from build123d import *

# Parameters (mm, degrees)
F1_DEPTH        = 1
F1_COPIES_COUNT = 10
F3_W            = 3
F3_H            = 3
F4_DEPTH        = 0.25
F5_DEPTH        = 1
F6_DEPTH        = 0.25
F7_R            = 1.1
F8_DEPTH        = 12.5


# Not quite as in the source:
# - ends of sketch curves that miss each other by under 0.0002 mm in the source are joined
# - a feature of the source that left no trace in its solid (it failed there, or was rolled back) is left out
# - a pattern or mirror of a feature is missing from the dataset's text; its kind, count and spacing are read off the source's solid


with BuildPart() as f1:
    # F0 (on Top) → F1 (new body)
    with BuildSketch(Plane.XY):
        with BuildLine():
            ThreePointArc((0.581444512, 2.1217733808), (0.2933415776, 2.1803556405), (0, 2.2))
            ThreePointArc((0, 2.2), (-0.2933416878, 2.1803556256), (-0.5814447265, 2.121773322))
            ThreePointArc((-0.5814447265, 2.121773322), (-0.5968372157, 2.1167523736), (-0.6125853979, 2.1129929319))
            ThreePointArc((-0.6125853979, 2.1129929319), (-1.3214219849, -1.7589326132), (2.2, 0))
            ThreePointArc((2.2, 0), (1.7589325969, 1.3214220066), (0.612585346, 2.112992947))
            ThreePointArc((0.6125853416, 2.1129929319), (0.5968370782, 2.1167523965), (0.581444512, 2.1217733808))
        make_face()
        with BuildLine():
            ThreePointArc((0.6, 0.8), (0, -1), (-0.6, 0.8))
            Line((-0.6, 0.8), (0, 0.8))
            Line((0, 0.8), (0.6, 0.8))
        make_face(mode=Mode.SUBTRACT)
        with BuildLine():
            ThreePointArc((-0.5814447265, 2.121773322), (-0.2933416878, 2.1803556256), (0, 2.2))
            Line((0, 2.2), (0, 2.8273255734))
            ThreePointArc((0, 2.8273255734), (-0.1215931939, 2.889819495), (-0.1419835484, 3.0250031792))
            Line((-0.1419835484, 3.0250031792), (-0.4660251262, 2.233467269))
            ThreePointArc((-0.4660251262, 2.233467269), (-0.5120300634, 2.1655250062), (-0.5814447265, 2.121773322))
        make_face()
        with BuildLine():
            Line((0, 2.8273255734), (0, 2.2))
            ThreePointArc((0, 2.2), (0.2933415776, 2.1803556405), (0.581444512, 2.1217733808))
            ThreePointArc((0.581444512, 2.1217733808), (0.5119904355, 2.165563311), (0.4659834267, 2.2335690598))
            Line((0.4659834267, 2.2335690598), (0.1424618925, 3.0249932315))
            ThreePointArc((0.1424618925, 3.0249932315), (0.1482808399, 3.0014743175), (0.1502375048, 2.9773253853))
            ThreePointArc((0.1502375048, 2.9773253853), (0.1062195181, 2.8711754307), (0, 2.8273255734))
        make_face()
        with BuildLine():
            ThreePointArc((-0.1419835484, 3.0250031792), (-0.1215931939, 2.889819495), (0, 2.8273255734))
            Line((0, 2.8273255734), (0, 3.1273251973))
            ThreePointArc((0, 3.1273251973), (-0.0874611784, 3.0990173775), (-0.1419835484, 3.0250031792))
        make_face()
        with BuildLine():
            Line((0, 3.1273251973), (0, 2.8273255734))
            ThreePointArc((0, 2.8273255734), (0.1062195181, 2.8711754307), (0.1502375048, 2.9773253853))
            ThreePointArc((0.1502375048, 2.9773253853), (0.1482808399, 3.0014743175), (0.1424618925, 3.0249932315))
            ThreePointArc((0.1424618925, 3.0249932315), (0.0877476558, 3.0991530237), (0, 3.1273251973))
        make_face()
        with BuildLine():
            ThreePointArc((0.612585346, 2.112992947), (0.5970310708, 2.1174404125), (0.581444512, 2.1217733808))
            ThreePointArc((0.581444512, 2.1217733808), (0.5968370782, 2.1167523965), (0.6125853416, 2.1129929319))
        make_face()
        with BuildLine():
            ThreePointArc((-0.6125853979, 2.1129929319), (-0.5968372157, 2.1167523736), (-0.5814447265, 2.121773322))
            ThreePointArc((-0.5814447265, 2.121773322), (-0.5970312038, 2.117440375), (-0.6125853979, 2.1129929319))
        make_face()
    extrude(amount=F1_DEPTH)

    # F1_copies: F1 ×10 about axis
    f1_copies_axis = Axis((0, 0, 0), (0, 0, 1))


with BuildPart() as f1_1:
    add(f1.part)
    for i in range(1, F1_COPIES_COUNT):
        add(f1.part.rotate(f1_copies_axis, i * 360 / F1_COPIES_COUNT))

    # F3 (on face) → F4 (cut)
    with BuildSketch(Plane.XY.offset(1)):
        Rectangle(F3_W, F3_H)
    extrude(amount=-F4_DEPTH, mode=Mode.SUBTRACT)

    # F0 (on Top) → F5 (join)
    with BuildSketch(Plane.XY):
        with BuildLine():
            ThreePointArc((0.581444512, 2.1217733808), (0.2933415776, 2.1803556405), (0, 2.2))
            ThreePointArc((0, 2.2), (-0.2933416878, 2.1803556256), (-0.5814447265, 2.121773322))
            ThreePointArc((-0.5814447265, 2.121773322), (-0.5968372157, 2.1167523736), (-0.6125853979, 2.1129929319))
            ThreePointArc((-0.6125853979, 2.1129929319), (-1.3214219849, -1.7589326132), (2.2, 0))
            ThreePointArc((2.2, 0), (1.7589325969, 1.3214220066), (0.612585346, 2.112992947))
            ThreePointArc((0.6125853416, 2.1129929319), (0.5968370782, 2.1167523965), (0.581444512, 2.1217733808))
        make_face()
        with BuildLine():
            ThreePointArc((0.6, 0.8), (0, -1), (-0.6, 0.8))
            Line((-0.6, 0.8), (0, 0.8))
            Line((0, 0.8), (0.6, 0.8))
        make_face(mode=Mode.SUBTRACT)
        with BuildLine():
            ThreePointArc((-0.5814447265, 2.121773322), (-0.2933416878, 2.1803556256), (0, 2.2))
            Line((0, 2.2), (0, 2.8273255734))
            ThreePointArc((0, 2.8273255734), (-0.1215931939, 2.889819495), (-0.1419835484, 3.0250031792))
            Line((-0.1419835484, 3.0250031792), (-0.4660251262, 2.233467269))
            ThreePointArc((-0.4660251262, 2.233467269), (-0.5120300634, 2.1655250062), (-0.5814447265, 2.121773322))
        make_face()
        with BuildLine():
            Line((0, 2.8273255734), (0, 2.2))
            ThreePointArc((0, 2.2), (0.2933415776, 2.1803556405), (0.581444512, 2.1217733808))
            ThreePointArc((0.581444512, 2.1217733808), (0.5119904355, 2.165563311), (0.4659834267, 2.2335690598))
            Line((0.4659834267, 2.2335690598), (0.1424618925, 3.0249932315))
            ThreePointArc((0.1424618925, 3.0249932315), (0.1482808399, 3.0014743175), (0.1502375048, 2.9773253853))
            ThreePointArc((0.1502375048, 2.9773253853), (0.1062195181, 2.8711754307), (0, 2.8273255734))
        make_face()
        with BuildLine():
            ThreePointArc((-0.1419835484, 3.0250031792), (-0.1215931939, 2.889819495), (0, 2.8273255734))
            Line((0, 2.8273255734), (0, 3.1273251973))
            ThreePointArc((0, 3.1273251973), (-0.0874611784, 3.0990173775), (-0.1419835484, 3.0250031792))
        make_face()
        with BuildLine():
            Line((0, 3.1273251973), (0, 2.8273255734))
            ThreePointArc((0, 2.8273255734), (0.1062195181, 2.8711754307), (0.1502375048, 2.9773253853))
            ThreePointArc((0.1502375048, 2.9773253853), (0.1482808399, 3.0014743175), (0.1424618925, 3.0249932315))
            ThreePointArc((0.1424618925, 3.0249932315), (0.0877476558, 3.0991530237), (0, 3.1273251973))
        make_face()
        with BuildLine():
            ThreePointArc((0.612585346, 2.112992947), (0.5970310708, 2.1174404125), (0.581444512, 2.1217733808))
            ThreePointArc((0.581444512, 2.1217733808), (0.5968370782, 2.1167523965), (0.6125853416, 2.1129929319))
        make_face()
        with BuildLine():
            ThreePointArc((-0.6125853979, 2.1129929319), (-0.5968372157, 2.1167523736), (-0.5814447265, 2.121773322))
            ThreePointArc((-0.5814447265, 2.121773322), (-0.5970312038, 2.117440375), (-0.6125853979, 2.1129929319))
        make_face()
    extrude(amount=F5_DEPTH)

    # F3 (on face) → F6 (join)
    with BuildSketch(Plane.XY.offset(1)):
        Rectangle(F3_W, F3_H)
        Polygon((-0.259935757, 0.8), (0.259935757, 0.8), (0.6805206467, 0.494427191), (0.8411697794, 0), (0.6805206467, -0.494427191), (0.259935757, -0.8), (-0.259935757, -0.8), (-0.6805206467, -0.494427191), (-0.8411697794, 0), (-0.6805206467, 0.494427191), align=None, mode=Mode.SUBTRACT)
    extrude(amount=F6_DEPTH)

    # F7 (on face) → F8 (cut, symmetric)
    with BuildSketch(Plane.XY.offset(1)):
        Circle(F7_R)
    extrude(amount=F8_DEPTH, both=True, mode=Mode.SUBTRACT)


solid = f1_1.part
Could you check a few things on this model? Use its own coordinates, in mm. A direction names the side the tool comes from. Give positions to 0.01 mm unless a question says otherwise; leave off trailing zeros. Order: outer loops, then holes, each group sorted by start corner. A loop starts at its lowest first (then second) coordinate and runs counter-clockwise, first axis right, second up. Notation, with made-up numbers: (49, 68) -> (96, 68) arc R11 ccw to (96, 81) -> close; hole circle Ø9 at (56, -28). An arc over 180 degrees is marked (long way). Return JSON: item names as keys, results as strings.
1. Thinking about a two-plate mould opening in Y: for faces 4 (the flat face through (2.41, 1.1, 0.49)), 5 (the flat face through (-1, -1, 0)), 6 (the flat face through (-1.79, -1.94, 0.49)), which applies, pulls with the +Y half, pulls with the -Y half, needs draft (parallel to the pull), parting line crosses it, or undercut?
Answer list:
{"face 4": "pulls with the +Y half", "face 5": "needs draft", "face 6": "undercut"}
2. Imagine slicing it at A-A on x = 2.6. List the corners of the cut face in (y, z) for me, then the cut area to 3 significant figures.
Answer list:
{"outline": "(-1.09, 0) -> (-0.53, 0) -> (-0.53, 1) -> (-1.09, 1) -> close; (0.53, 0) -> (1.09, 0) -> (1.09, 1) -> (0.53, 1) -> close", "area": "1.12 mm2"}
3. For pin 1 Ø1.8 at (x, y) = (0, 0) entering from -Z, with a flat end and sliding along its axis, tell me the tip position at first contact or that it passes through.
Answer list:
{"pin 1": "passes through"}
4. Imagine slicing it at B-B on y = 2.75. List the corners of the cut face in (x, z) for me.
Answer list:
{"outline": "(-0.25, 0) -> (0.25, 0) -> (0.25, 1) -> (-0.25, 1) -> close"}
5. On a 3-axis mill with a long thin cutter (end or side, diameter ignored), from which of +Z, -Z, +X, -X, +Y, -Y can I reach the whole of each face in a straight line? I mean faces 1 (the cylindrical face through (1.05, 0.33, 0.63)), 2 (the flat face through (1.79, -1.95, 0.49)), 3 (the flat face through (-1.79, 1.95, 0.49)). Say none if no direction works.
Answer list:
{"face 1": "+Z, -Z", "face 2": "+Z, -Z, +X", "face 3": "+Z, -Z, -X"}
6. I need wall thicknesses on line 1 (Y direction, x = 0, z = 0.7); line 2 (Y direction, x = 0, z = 1.05); line 3 (Y direction, x = 2, z = 0.5). Which ranges of each line are inside material? Lowest first, please. Write a range as from..to.
Answer list:
{"line 1": "y = -3.13..-1.1, 1.1..3.13", "line 2": "y = -1.5..-1.1, 1.1..1.5", "line 3": "y = -1.13..1.13"}
